Input: part model. Units: mm. Frame: model coordinates. A direction names the side the tool comes from. Round coordinates to 2 decimals unless told otherwise and drop trailing zeros. Write each loop counter-clockwise with the first axis right and the second up, starting at its lowest first coordinate (ties: lowest second). Pieces come first, ordered by that corner, then holes. Notation, with made-up numbers: (25, 39) -> (33, 39) arc R26 ccw to (33, 65) -> close; hole circle Ø10 at (70.25, 53). An arc over 180 degrees is marked (long way). Use CSV: the item, a comma, the result in double quotes.
Autodesk Fusion 360 part; units mm, degrees
sketch "Sketch1" plane through (0, 0, 0) normal (0, 0, 1) x (1, 0, 0)
  line L0 (-100, 50) -> (346.68, 50)
  line L1 (346.68, 50) -> (346.68, -116.26)
  line L2 (346.68, -116.26) -> (-100, -116.26)
  line L3 (-100, -116.26) -> (-100, 50)
  line L4 (-110, 60) -> (356.68, 60)
  line L5 (356.68, 60) -> (356.68, -126.26)
  line L6 (356.68, -126.26) -> (-110, -126.26)
  line L7 (-110, -126.26) -> (-110, 60)
  dimension "d1" = 446.68
  dimension "d2" = 166.26
  dimension "d3" = 466.68
  dimension "d4" = 186.26
  dimension "d5" = 10
  dimension "d6" = 10
extrude "Extrude1" add sketch "Sketch1" along normal blind 5 contours L0 L1 L2 L3
extrude "Extrude2" add sketch "Sketch1" along normal blind 18
sketch "Sketch2" plane through (0, 0, 5) normal (0, 0, 1) x (-1, 0, 0)
  line L0 (100, 116.26) -> (-346.68, 116.26)
  line L1 (-346.68, 116.26) -> (-346.68, -50)
  line L2 (-346.68, -50) -> (100, -50)
  line L3 (100, -50) -> (100, 116.26)
  circle A0 centre (94, -45.04) radius 1.7
  circle A1 centre (-132.22, -32.1) radius 1.7
  circle A2 centre (92.07, 82.66) radius 1.7
  circle A3 centre (-95.96, 112.43) radius 1.7
  circle A4 centre (-237.26, 64.33) radius 1.7
  circle A5 centre (-335.42, -43.13) radius 1.7
  circle A6 centre (-336.97, 108.98) radius 1.7
  line L4 (100, -50) -> (-346.68, -50)
  line L5 (100, 116.26) -> (100, -50)
  line L6 (-346.68, 116.26) -> (100, 116.26)
  line L7 (-346.68, -50) -> (-346.68, 116.26)
  dimension "d11" = 3.4
  dimension "d12" = 3.4
  dimension "d13" = 3.4
  dimension "d14" = 3.4
  dimension "d15" = 3.4
  dimension "d16" = 3.4
  dimension "d17" = 3.4
  dimension "d18" = 4.96
  dimension "d19" = 6
  dimension "d20" = 7.93
  dimension "d21" = 33.6
  dimension "d22" = 195.96
  dimension "d23" = 3.83
  dimension "d24" = 109.42
  dimension "d25" = 51.93
  dimension "d26" = 7.28
  dimension "d27" = 9.71
  dimension "d28" = 11.26
  dimension "d29" = 6.87
  dimension "d30" = 214.46
  dimension "d31" = 17.9
extrude "Extrude3" add sketch "Sketch2" along normal blind 8 contours A0 | A1 | A2 | A3 | A4 | A5 | A6
fillet "Fillet1" radius 5 4 edges at (356.68, -126.26, 9) (356.68, 60, 9) (-110, 60, 9) (-110, -126.26, 9)
Item 1: Section query B-B on x = 143. Return the cut outline in (y, z).
Worked answers:
outline,"(-126.26, 0) -> (60, 0) -> (60, 18) -> (50, 18) -> (50, 5) -> (-116.26, 5) -> (-116.26, 18) -> (-126.26, 18) -> close"
Item 2: Set-up query: faces 1 (the face through (356.68, -32, 9)), 2 (the face through (126, -116.26, 11)). Return all of +Z, -Z, +X, -X, +Y, -Y with unobstructed straight access to the full face (end or side cutting, diameter ignored); none if empty.
Worked answers:
face 1,"+Z, -Z, +X, +Y, -Y"
face 2,"+Z"
Item 3: Pull-direction query (Y, two-part tool) for faces 3 (the face through (120, -32, 5)), 4 (the face through (127, -126.26, 9)), 5 (the face through (120, 60, 9)); classes: +Y half, -Y half, draft (parallel to the pull), parting line (faces both ways), or undercut.
Worked answers:
face 3,"undercut"
face 4,"-Y half"
face 5,"+Y half"
Item 4: Line query: line 1 (X direction, y = -86.5, z = 5.5); line 2 (Y direction, x = 80.5, z = 16.5); line 3 (Z direction, x = -58, y = -115). Output: solid intervals per line, ascending.
Worked answers:
line 1,"x = -110 to -100, 346.68 to 356.68"
line 2,"y = -126.26 to -116.26, 50 to 60"
line 3,"z = 0 to 5"
Item 5: First-contact query: pin 1 Ø4 at (x, y) = (146, -90.5) entering from +Z; pin 2 Ø2.5 at (x, y) = (237, -64) entering from +Z. Flat tips, straight axial feed; report the tip coordinate or a pass-through.
Worked answers:
pin 1,"stops at z = 5"
pin 2,"stops at z = 13"
Item 6: Section query A-A on z = 8.5. Give the number of separate pieces and of enclosed holes in the cut face, plus the area to 3 significant figures.
Worked answers:
separate pieces,"8"
enclosed holes,"1"
area,"12,700 mm²"
Item 7: Section query C-C on y = -35. Return the cut outline in (x, z).
Worked answers:
outline,"(-110, 0) -> (356.68, 0) -> (356.68, 18) -> (346.68, 18) -> (346.68, 5) -> (-100, 5) -> (-100, 18) -> (-110, 18) -> close"
